Work out the finished part from the listing and answer in its coordinate system (mm). Round coordinates to 2 decimals unless told otherwise and drop trailing zeros. Loops run counter-clockwise (first coordinate to the right, second up) from the corner with the lowest first, then second, coordinate; pieces in that order, holes last. Notation, with made-up numbers: (-3.5, 22) - (9.5, 22) arc R9 ccw to (9.5, 37) - close; hole circle Ø1 at (26.25, 65.5). An arc over 180 degrees is marked (long way). Return JSON: item names as keys, results as strings.
from build123d import *

# Parameters (mm, degrees)
REVOLVE1_ANGLE     = 72
CUT_EXTRUDE2_DEPTH = 0.635
CUT_EXTRUDE3_DEPTH = 0.635
SKETCH2_R          = 12.7
CUT_EXTRUDE1_DEPTH = 25.4
CUT_EXTRUDE4_REACH = 151.001


with BuildPart() as part:
    # Sketch1 → Revolve1 (revolve)
    with BuildSketch(Plane.XY):
        with BuildLine():
            Line((0, 0), (0, 76.2))
            Line((0, 76.2), (88.9, 76.2))
            ThreePointArc((88.9, 76.2), (98.376882891, 51.581720723), (101.6, 25.4))
            Line((101.6, 25.4), (101.6, 0))
            Line((101.6, 0), (0, 0))
        make_face()
    revolve(axis=Axis((0, 0, 0), (0, 1, 0)), revolution_arc=REVOLVE1_ANGLE)

    # Sketch3 → Cut-Extrude2 (cut)
    with BuildSketch(Plane(origin=(0, 0, 0), x_dir=(-0.3090169943749449, 0, 0.9510565162951544), z_dir=(-0.9510565162951544, 0, -0.3090169943749449))):
        with BuildLine():
            Line((0, 76.2), (-88.9, 76.2))
            ThreePointArc((-88.9, 76.2), (-98.376882891, 51.581720723), (-101.6, 25.4))
            Line((-101.6, 25.4), (-101.6, 0))
            Line((-101.6, 0), (0, 0))
            Line((0, 0), (0, 76.2))
        make_face()
    extrude(amount=-CUT_EXTRUDE2_DEPTH, mode=Mode.SUBTRACT)

    # Sketch4 → Cut-Extrude3 (cut)
    with BuildSketch(Plane.XY):
        with BuildLine():
            Line((0.667678512, 76.2), (0.667678512, 0))
            Line((0.667678512, 0), (101.6, 0))
            Line((101.6, 0), (101.6, 25.4))
            ThreePointArc((101.6, 25.4), (98.376882891, 51.581720723), (88.9, 76.2))
            Line((88.9, 76.2), (0.667678512, 76.2))
        make_face()
    extrude(amount=-CUT_EXTRUDE3_DEPTH, mode=Mode.SUBTRACT)

    # Sketch2 → Cut-Extrude1 (cut)
    with BuildSketch(Plane(origin=(0, 76.2, 0), x_dir=(1, 0, 0), z_dir=(0, 1, 0))):
        Circle(SKETCH2_R)
    extrude(amount=-CUT_EXTRUDE1_DEPTH, mode=Mode.SUBTRACT)

    # Sketch5 → Cut-Extrude4 (cut, up to next)
    with BuildSketch(Plane(origin=(0, 50.8, 0), x_dir=(1, 0, 0), z_dir=(0, 1, 0)), mode=Mode.PRIVATE) as cut_extrude4_sk1:
        Polygon((1.658905685, 0.635), (1.116550937, 1.38148727), (0.874002519, 0.635), align=None)
    cut_extrude4_tool1 = extrude(cut_extrude4_sk1.sketch, amount=-CUT_EXTRUDE4_REACH, mode=Mode.PRIVATE) & part.part
    add(cut_extrude4_tool1.solids().sort_by_distance((1.216486, 50.8, -0.883829))[0], mode=Mode.SUBTRACT)


solid = part.part
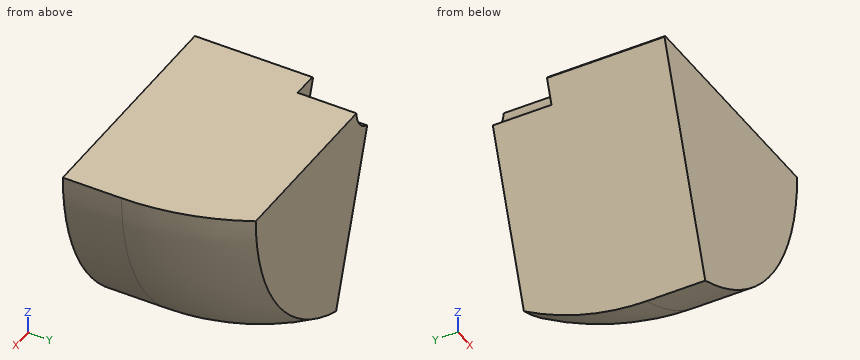
1) Section A-A (x = 15.5) is taken. Give the vertices of the cut face in (y, z) (3 decimals), and give its area (3 significant figures).
Verdict:
{"outline": "(0, -45.649) - (76.2, -45.649) - (76.2, -0.635) - (0, -0.635) - close", "area": "3,430 mm2"}
2) Flat-ended cylindrical pins translate along their axes: pin 1 (5 mm diameter, centred on y = 56.5, z = -74.5, fed in from -X); pin 2 (10 mm diameter, centred on y = 48, z = -80, fed in from +X); pin 3 (12 mm diameter, centred on y = 18.5, z = -20, fed in from -X). Find the tip coordinate at first contact, or state that the pin passes through.
Verdict:
{"pin 1": "stops at x = 24.06", "pin 2": "stops at x = 65.15", "pin 3": "stops at x = 5.22"}
3) Find the intervals of material crossed by L1, parallel to X at y = 54, z = -18.5; L2, parallel to X at y = 56, z = -39; L3, parallel to Z at x = 61.5, y = 41 (3 decimals), in increasing order.
Verdict:
{"L1": "x = 6.68 to 95.98", "L2": "x = 13.34 to 89", "L3": "z = -79.444 to -0.635"}
